Verification items for this drawing (mm, ordinates from the low corner). A direction names the side the tool comes from. Give positions to 0.01 mm unless a question says otherwise; leave off trailing zeros. Write each loop counter-clockwise with the first axis right and the second up, starting at its lowest first coordinate (ties: lowest second). Pieces come first, ordered by that corner, then holes. Notation, with made-up numbers: (-29, 17.5) -> (2, 17.5) arc R7 cw to (2, 28.5) -> close; hole circle Ø5 at (-29, 35.5). An arc over 180 degrees is marked (long way). Answer as a JSON object with one key per item and string values.
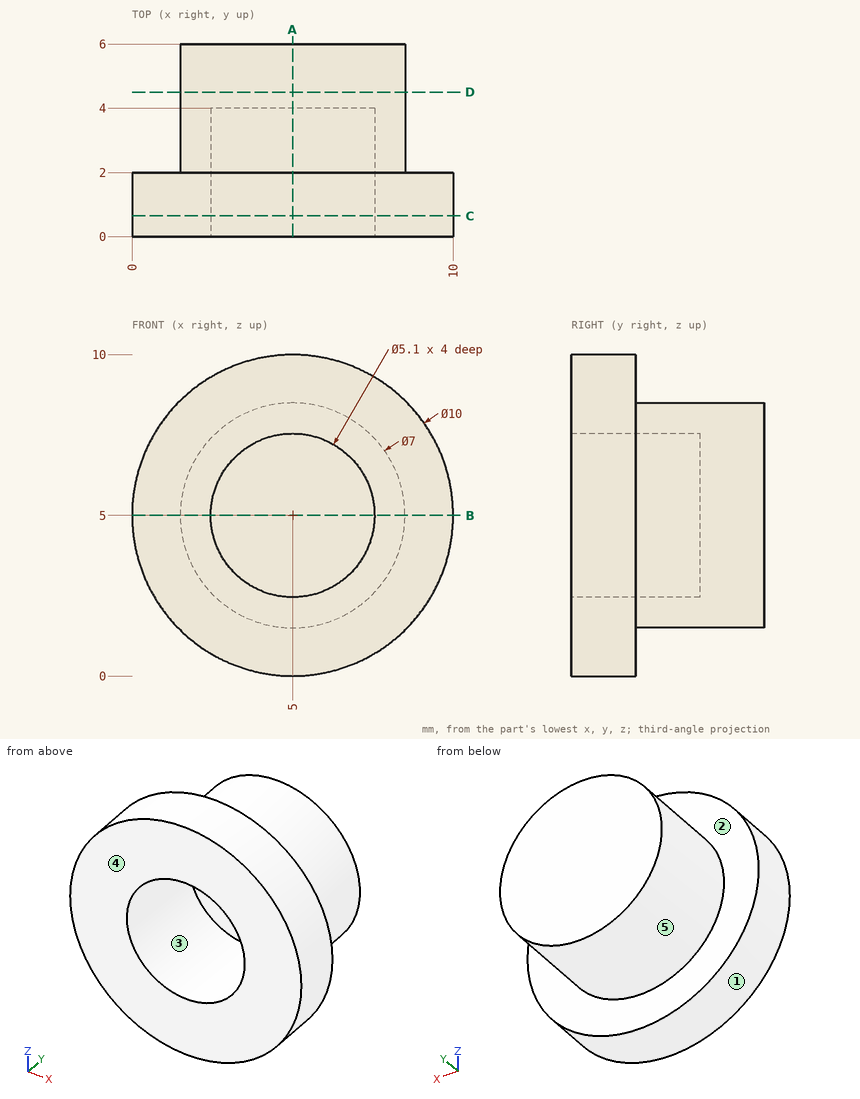
1. Scan lines: L1, parallel to X at y = 1.7, z = 5; L2, parallel to X at y = 2.15, z = 5; L3, parallel to Y at x = 3.5, z = 4. Record each from-to range of solid material in increasing order. Write a range as [from, to].
Determined:
{"L1": "[0, 2.45], [7.55, 10]", "L2": "[1.5, 2.45], [7.55, 8.5]", "L3": "[4, 6]"}
2. Sectioned sample at B-B, the plane z = 5. Enter the section's corners in (x, y), plus the area to 3 significant figures.
Determined:
{"outline": "(0, 0) -> (2.45, 0) -> (2.45, 4) -> (7.55, 4) -> (7.55, 0) -> (10, 0) -> (10, 2) -> (8.5, 2) -> (8.5, 6) -> (1.5, 6) -> (1.5, 2) -> (0, 2) -> close", "area": "27.6 mm^2"}
3. Sectioned sample at C-C, the plane y = 0.65. Enter the section's corners in (x, z).
Determined:
{"outline": "circle Ø10 at (5, 5); hole circle Ø5.1 at (5, 5)"}
4. Access from +Z, -Z, +X, -X, +Y, -Y to the whole of each face (thin tool, end or side, straight path). Record for the marked faces 1 and 2.
Determined:
{"face 1": "+Y, -Y", "face 2": "+Y"}
5. Go/stop test with a flat-tipped pin: P1, Ø2.5, axis at x = 5.5, z = 4.5, coming from the -Y side. Record where the tip stops, or that it passes through.
Determined:
{"P1": "y = 4"}
6. Mould release check, pull along X, two halves, no side actions. Record for the marked faces 3, 4 and 5: released by +X, released by -X, zero draft, split by the parting line, or undercut.
Determined:
{"face 3": "undercut", "face 4": "zero draft", "face 5": "split by the parting line"}
7. Sectioned sample at D-D, the plane y = 4.5. Enter the section's corners in (x, z).
Determined:
{"outline": "circle Ø7 at (5, 5)"}
8. Sectioned sample at A-A, the plane x = 5. Enter the section's corners in (y, z).
Determined:
{"outline": "(0, 0) -> (2, 0) -> (2, 1.5) -> (6, 1.5) -> (6, 8.5) -> (2, 8.5) -> (2, 10) -> (0, 10) -> (0, 7.55) -> (4, 7.55) -> (4, 2.45) -> (0, 2.45) -> close"}
